Check sheet for the modelled part. Datum: model origin and axes. Units: mm. Face numbers are marked on the shaded views. A direction names the side the tool comes from. Round coordinates to 2 decimals unless told otherwise and drop trailing zeros. Write each loop counter-clockwise with the first axis right and the second up, starting at its lowest first coordinate (ties: lowest second). Pieces come first, ordered by that corner, then holes. Notation, with made-up numbers: M 33.5,14 L 72.5,14 A26 cw 72.5,49 Z; hole C 4.5,19 d10. An arc over 180 degrees is marked long. One line per item, written item: value.
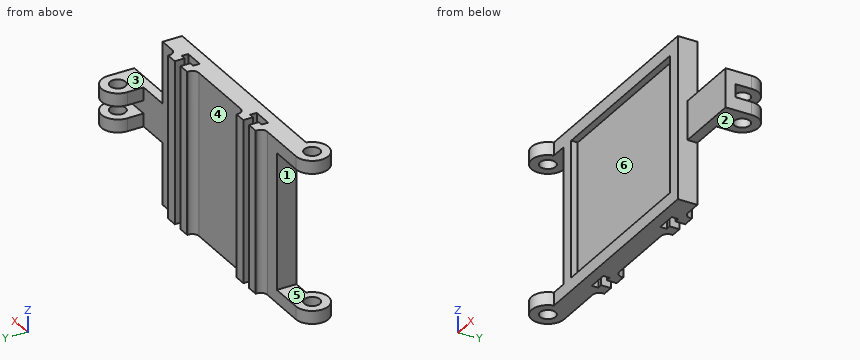
from build123d import *

# Parameters (mm, degrees)
ESBO_O1_W                         = 300
ESBO_O1_H                         = 250
RESSALTO_EXTRUS_O1_DEPTH          = 30
ESBO_O3_W                         = 50
ESBO_O3_H                         = 250
RESSALTO_EXTRUS_O2_DEPTH          = 12
FILETE1_R                         = 10
CORTE_EXTRUS_O1_REACH             = 127
CORTE_EXTRUS_O1_DIRECTION_2_REACH = 127
ESBO_O5_R                         = 12
RESSALTO_EXTRUS_O3_DEPTH          = 30
ESBO_O6_W                         = 60.214883571
ESBO_O6_H                         = 66.59752961
CORTE_EXTRUS_O2_DEPTH             = 10
ESBO_O7_R                         = 12
RESSALTO_EXTRUS_O4_DEPTH          = 20
ESBO_O8_W                         = 260
ESBO_O8_H                         = 210
CORTE_EXTRUS_O3_DEPTH             = 10


with BuildPart() as part:
    # Esboço1 → Ressalto-extrusão1 (new body)
    with BuildSketch(Plane(origin=(0, 0, 0), x_dir=(1, 0, 0), z_dir=(0, 1, 0))):
        Rectangle(ESBO_O1_W, ESBO_O1_H)
    extrude(amount=RESSALTO_EXTRUS_O1_DEPTH)

    # Esboço3 → Ressalto-extrusão2 (add)
    with BuildSketch(Plane(origin=(0, 30, 0), x_dir=(1, 0, 0), z_dir=(0, 1, 0))):
        with Locations((90, 0)):
            Rectangle(ESBO_O3_W, ESBO_O3_H)
        with Locations((-90, 0)):
            Rectangle(ESBO_O3_W, ESBO_O3_H)
    extrude(amount=RESSALTO_EXTRUS_O2_DEPTH)

    # Filete1
    filete1_edges = [part.edges().sort_by_distance(p)[0] for p in [
        (-115, 30, 0),
        (-65, 30, 0),
        (65, 30, 0),
        (115, 30, 0),
    ]]
    fillet(filete1_edges, radius=FILETE1_R)

    # Esboço4 → Corte-extrusão1 (cut, up to next)
    with BuildSketch(Plane.XY, mode=Mode.PRIVATE) as corte_extrus_o1_sk1:
        Polygon((82.5, 42), (97.5, 42), (97.5, 27), (105, 27), (105, 17), (75, 17), (75, 27), (82.5, 27), align=None)
    corte_extrus_o1_tool1 = extrude(corte_extrus_o1_sk1.sketch, amount=-CORTE_EXTRUS_O1_REACH, mode=Mode.PRIVATE) & part.part
    add(corte_extrus_o1_tool1.solids().sort_by_distance((90, 27.357143, 0))[0], mode=Mode.SUBTRACT)
    # Esboço4 → Corte-extrusão1 (cut, up to next)
    with BuildSketch(Plane.XY, mode=Mode.PRIVATE) as corte_extrus_o1_sk2:
        Polygon((-82.5, 42), (-82.5, 27), (-75, 27), (-75, 17), (-105, 17), (-105, 27), (-97.5, 27), (-97.5, 42), align=None)
    corte_extrus_o1_tool2 = extrude(corte_extrus_o1_sk2.sketch, amount=-CORTE_EXTRUS_O1_REACH, mode=Mode.PRIVATE) & part.part
    add(corte_extrus_o1_tool2.solids().sort_by_distance((-90, 27.357143, 0))[0], mode=Mode.SUBTRACT)

    # Esboço4 → Corte-extrusão1 direction 2 (cut, up to next)
    with BuildSketch(Plane.XY, mode=Mode.PRIVATE) as corte_extrus_o1_direction_2_sk1:
        Polygon((82.5, 42), (97.5, 42), (97.5, 27), (105, 27), (105, 17), (75, 17), (75, 27), (82.5, 27), align=None)
    corte_extrus_o1_direction_2_tool1 = extrude(corte_extrus_o1_direction_2_sk1.sketch, amount=CORTE_EXTRUS_O1_DIRECTION_2_REACH, mode=Mode.PRIVATE) & part.part
    add(corte_extrus_o1_direction_2_tool1.solids().sort_by_distance((90, 27.357143, 0))[0], mode=Mode.SUBTRACT)
    # Esboço4 → Corte-extrusão1 direction 2 (cut, up to next)
    with BuildSketch(Plane.XY, mode=Mode.PRIVATE) as corte_extrus_o1_direction_2_sk2:
        Polygon((-82.5, 42), (-82.5, 27), (-75, 27), (-75, 17), (-105, 17), (-105, 27), (-97.5, 27), (-97.5, 42), align=None)
    corte_extrus_o1_direction_2_tool2 = extrude(corte_extrus_o1_direction_2_sk2.sketch, amount=CORTE_EXTRUS_O1_DIRECTION_2_REACH, mode=Mode.PRIVATE) & part.part
    add(corte_extrus_o1_direction_2_tool2.solids().sort_by_distance((-90, 27.357143, 0))[0], mode=Mode.SUBTRACT)

    # Esboço5 → Ressalto-extrusão3 (add, symmetric)
    with BuildSketch(Plane.XY):
        with BuildLine():
            Line((150, 30), (200, 30))
            Line((200, 30), (200, 55))
            ThreePointArc((200, 55), (225, 80), (250, 55))
            Line((250, 55), (250, 15))
            Line((250, 15), (150, 15))
            Line((150, 15), (150, 30))
        make_face()
        with Locations((225, 55)):
            Circle(ESBO_O5_R, mode=Mode.SUBTRACT)
    extrude(amount=RESSALTO_EXTRUS_O3_DEPTH, both=True)

    # Esboço6 → Corte-extrusão2 (cut, symmetric)
    with BuildSketch(Plane.XY):
        with Locations((230.107441786, 63.298764805)):
            Rectangle(ESBO_O6_W, ESBO_O6_H)
    extrude(amount=CORTE_EXTRUS_O2_DEPTH, both=True, mode=Mode.SUBTRACT)

    # Esboço7 → Ressalto-extrusão4 (add)
    with BuildSketch(Plane.XY.offset(125)):
        with BuildLine():
            Line((-150, 30), (-200, 30))
            ThreePointArc((-200, 30), (-219.364916731, -10.811388301), (-175.505102572, 0))
            Line((-175.505102572, 0), (-150, 0))
            Line((-150, 0), (-150, 30))
        make_face()
        with Locations((-200, 5)):
            Circle(ESBO_O7_R, mode=Mode.SUBTRACT)
    ressalto_extrus_o4 = extrude(amount=-RESSALTO_EXTRUS_O4_DEPTH)

    # Espelhar1: Ressalto-extrusão4 across plane
    add(ressalto_extrus_o4.mirror(Plane.XY))

    # Esboço8 → Corte-extrusão3 (cut)
    with BuildSketch(Plane.XZ):
        Rectangle(ESBO_O8_W, ESBO_O8_H)
    extrude(amount=-CORTE_EXTRUS_O3_DEPTH, mode=Mode.SUBTRACT)


solid = part.part
Q1. Access from +Z, -Z, +X, -X, +Y, -Y to the whole of each face (thin tool, end or side, straight path). Record for the marked faces 4, 5 and 6.
Completed:
face 4: +Z, -Z, +Y
face 5: -X, +Y, -Y
face 6: -Y
Q2. Sectioned sample at B-B on y = 5. Enter the section's corners in (x, z), and give its area (3 significant figures).
Completed:
outline: M -225,-125 L -212,-125 L -212,-105 L -225,-105 Z; M -225,105 L -212,105 L -212,125 L -225,125 Z; M -188,-125 L 150,-125 L 150,125 L -188,125 L -188,105 L -150,105 L -150,-105 L -188,-105 Z; hole M -130,-105 L 130,-105 L 130,105 L -130,105 Z
area: 22,400 mm^2
Q3. Sectioned sample at A-A on x = 225. Enter the section's corners in (y, z).
Completed:
outline: M 15,-30 L 43,-30 L 43,-10 L 30,-10 L 30,10 L 43,10 L 43,30 L 15,30 Z; M 67,-30 L 80,-30 L 80,-10 L 67,-10 Z; M 67,10 L 80,10 L 80,30 L 67,30 Z
Q4. Depth check by flat-ended pin: P1, Ø2, axis at x = 80, z = -49, coming from the -Y side; P2, Ø10, axis at x = -131.5, z = 22.5, coming from the -Y side; P3, Ø3, axis at y = 21, z = 7.5, coming from the -X side. Enter the tip coordinate at first touch or a pass-through.
Completed:
P1: y = 10
P2: y = 0
P3: x = -150
Q5. Draft check along Z on the marked faces 1, 2 and 3. Enter one of: pulls with the +Z half, pulls with the -Z half, needs draft (parallel to the pull), parting line crosses it, or undercut.
Completed:
face 1: undercut
face 2: pulls with the -Z half
face 3: pulls with the +Z half
Q6. Sectioned sample at C-C on x = -21. Enter the section's corners in (y, z), and give its area (3 significant figures).
Completed:
outline: M 0,-125 L 30,-125 L 30,125 L 0,125 L 0,105 L 10,105 L 10,-105 L 0,-105 Z
area: 5,400 mm^2
Q7. Scan lines: line 1 (X direction, y = 18, z = -71.5); line 2 (X direction, y = 55, z = -22); line 3 (Y direction, x = -200, z = 110.5). Record each from-to range of solid material in increasing order. Write a range as [from, to].
Completed:
line 1: [-150, -105], [-75, 75], [105, 150]
line 2: [200, 213], [237, 250]
line 3: [-20, -7], [17, 30]
